Verification items for the finished model (mm, model axes). A direction names the side the tool comes from. Round coordinates to 2 decimals unless told otherwise and drop trailing zeros. Write each loop counter-clockwise with the first axis right and the second up, starting at its lowest first coordinate (ties: lowest second). Pieces come first, ordered by that corner, then holes. Notation, with made-up numbers: M 31.25,62 L 78.25,62 A18 cw 78.25,90 Z; hole C -34,69 d10. An arc over 180 degrees is marked long. One line per item, written item: value. Start each with the question number.
Item 1: Draft check along Z on faces 4 (the face through (12.017, -15.042, -4.76)), 5 (the face through (-15.983, -15.042, -4.76)), 6 (the face through (-9, -6, -4)), 7 (the face through (0, -7, -9)). Enter one of: +Z half, -Z half, draft (parallel to the pull), parting line (faces both ways), or undercut.
Item 2: Gauge pin test, flat ends, axial feed: pin 1 (2 mm diameter, centred on y = -9.5, z = -1, fed in from +X); pin 2 (5 mm diameter, centred on x = 14, z = -4.5, fed in from +Y); pin 3 (1.5 mm diameter, centred on y = -2.5, z = -6, fed in from -X). Record the tip position at first contact, or that the pin passes through.
Item 3: Thickness scan on probe 1 along X at (y, z) = (-15.85, -4.5); probe 2 along Y at (x, z) = (0, -5.5); probe 3 along Z at (x, y) = (-14, -13.3). Record the ranges inside material, lowest first. Write a range as from..to.
Item 4: Section check A-A, the plane x = 0. Record the cut outline in (y, z).
Item 5: Section check B-B, the plane z = -4.5. Record the cut outline in (x, y), then the cut area to 3 significant figures.
Item 6: Section check D-D, the plane y = -7.25. Record the cut outline in (x, z).
Item 7: Tool access check on faces 1 (the face through (9, -6, -4)), 2 (the face through (0, -18, -4)), 3 (the face through (-12, -12, -3)). Record the directions out of +Z, -Z, +X, -X, +Y, -Y that give a thin tool (end or side, any length) a straight path to the whole face; none if there is none.
Item 8: Section check C-C, the plane z = -7. Record the cut outline in (x, y).
Autodesk Inventor part; units mm, degrees
ref_plane "YZ Plane" through (0, 0, 0) normal (1, 0, 0) x (0, 1, 0)
ref_plane "XZ Plane" through (0, 0, 0) normal (0, 1, 0) x (-1, 0, 0)
ref_plane "XY Plane" through (0, 0, 0) normal (0, 0, 1) x (1, 0, 0)
sketch "Sketch1" plane through (0, 0, 0) normal (0, 0, 1) x (1, 0, 0)
  circle A0 centre (0, 0) radius 4.5
  arc A1 (9, 0) -> (-9, 0) centre (0, 0) ccw
  line L0 (0, 0) -> (0, -47) construction
  line L1 (0, -18) -> (-18, -18)
  line L2 (0, -18) -> (18, -18)
  line L3 (18, -18) -> (18, -12)
  line L4 (18, -12) -> (10, -12)
  line L5 (9, -11) -> (9, 0)
  line L6 (-18, -18) -> (-18, -12)
  line L7 (-18, -12) -> (-10, -12)
  line L8 (-9, -11) -> (-9, 0)
  arc A2 (-10, -12) -> (-9, -11) centre (-10, -11) ccw
  arc A3 (9, -11) -> (10, -12) centre (10, -11) ccw
  dimension "d0" = 9
  dimension "d1" = 18
  dimension "d6" = 6
  dimension "d7" = 6
  dimension "d9" = 18
  dimension "d10" = 2
  dimension "d11" = 2
  dimension "d12" = 9
  dimension "d13" = 9
  dimension "d14" = 36
  dimension "d15" = 18
extrude "Extrusion1" add sketch "Sketch1" against normal blind 9 contours A0 | L5 A3 L4 L3 L2 L1 L6 L7 A2 L8 A1
hole "Hole1" at (0, 0, 0) direction (0, 0, -1) diameter 9 end through all
sketch "Sketch2" plane through (-18, -12, 0) normal (0, 1, 0) x (1, 0, 0)
  circle A0 centre (4, 4.5) radius 2
  circle A1 centre (32, 4.5) radius 2
  line L0 (8, 0) -> (0, 0)
  line L1 (0, 0) -> (0, 9)
  line L2 (36, 0) -> (28, 0)
  line L3 (36, 0) -> (36, 9)
  point P0 (18, 0)
  dimension "d25" = 4
  dimension "d26" = 4
  dimension "d27" = 4.5
  dimension "d28" = 4
  dimension "d29" = 4.5
  dimension "d30" = 4
hole "Hole2" at (-14, -12, -4.5) at (14, -12, -4.5) direction (0, -1, 0) diameter 4 end through all
fillet "Fillet1" radius 0.25 24 edges at (9, -5.5, -9) (9.2929, -11.7071, -9) (14, -12, -9) (-9, -5.5, -9) (-9.2929, -11.7071, -9) (-14, -12, -9) (0, 9, -9) (-9, -5.5, 0) (-9.2929, -11.7071, 0) (-14, -12, 0) (9, -5.5, 0) (9.2929, -11.7071, 0) (14, -12, 0) (0, 9, 0) (18, -12, -4.5) (-18, -12, -4.5) (18, -18, -4.5) (18, -15, -9) (18, -15, 0) (-18, -18, -4.5) (-18, -15, 0) (-18, -15, -9) (0, -18, -9) (0, -18, 0)
properties part number "HUDSON 1-04-REAR DRAWBAR BEAM BRACKET"
Response values:
1. face 4: undercut
1. face 5: undercut
1. face 6: draft
1. face 7: -Z half
2. pin 1: stops at x = 9
2. pin 2: stops at y = -12
2. pin 3: stops at x = -9
3. probe 1: x = -18..-16, -12..12, 16..18
3. probe 2: y = -18..-4.5, 4.5..9
3. probe 3: z = -9..-6.5, -2.5..0
4. outline: M -18,-8.75 A0.25 ccw -17.75,-9 L -4.5,-9 L -4.5,0 L -17.75,0 A0.25 ccw -18,-0.25 Z; M 4.5,-9 L 8.75,-9 A0.25 ccw 9,-8.75 L 9,-0.25 A0.25 ccw 8.75,0 L 4.5,0 Z
5. outline: M -18,-17.75 A0.25 ccw -17.75,-18 L -16,-18 L -16,-12 L -17.75,-12 A0.25 ccw -18,-12.25 Z; M -12,-18 L 12,-18 L 12,-12 L 10,-12 A1 cw 9,-11 L 9,0 A9 ccw -9,0 L -9,-11 A1 cw -10,-12 L -12,-12 Z; M 16,-18 L 17.75,-18 A0.25 ccw 18,-17.75 L 18,-12.25 A0.25 ccw 17.75,-12 L 16,-12 Z; hole C 0,0 d9
5. area: 448 mm2
6. outline: M -9,-8.75 A0.25 ccw -8.75,-9 L 8.75,-9 A0.25 ccw 9,-8.75 L 9,-0.25 A0.25 ccw 8.75,0 L -8.75,0 A0.25 ccw -9,-0.25 Z
7. face 1: +Z, -Z, +X, +Y
7. face 2: +Z, -Z, +X, -X, -Y
7. face 3: +Z, -Z, -X, +Y
8. outline: M -18,-17.75 A0.25 ccw -17.75,-18 L 17.75,-18 A0.25 ccw 18,-17.75 L 18,-12.25 A0.25 ccw 17.75,-12 L 10,-12 A1 cw 9,-11 L 9,0 A9 ccw -9,0 L -9,-11 A1 cw -10,-12 L -17.75,-12 A0.25 ccw -18,-12.25 Z; hole C 0,0 d9
